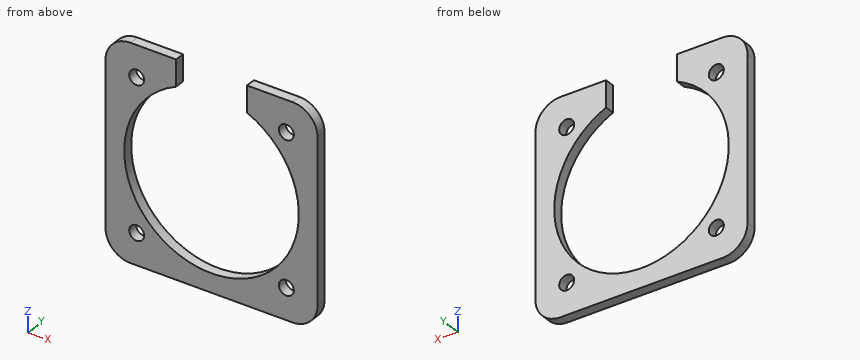
from build123d import *

# Parameters (mm, degrees)
SKETCH1_W           = 40.5
SKETCH1_H           = 40.5
SKETCH1_R           = 17.5
BOSS_EXTRUDE1_DEPTH = 2
SKETCH2_R           = 1.25
CUT_EXTRUDE1_DEPTH  = 2
CUT_EXTRUDE2_DEPTH  = 2
SKETCH4_W           = 42.5
SKETCH4_H           = 42.5
SKETCH4_W_2         = 40.5
SKETCH4_H_2         = 40.5
BOSS_EXTRUDE2_DEPTH = 2
SKETCH5_W           = 14.2
SKETCH5_H           = 2
CUT_EXTRUDE3_DEPTH  = 2
SKETCH6_R           = 1.5
CUT_EXTRUDE4_DEPTH  = 3.5
SKETCH7_R           = 1.5
BOSS_EXTRUDE3_DEPTH = 2
SKETCH8_R           = 1.5
CUT_EXTRUDE5_DEPTH  = 2
FILLET2_R           = 5


with BuildPart() as part:
    # Sketch1 → Boss-Extrude1 (new body)
    with BuildSketch(Plane(origin=(0, 0, 0), x_dir=(1, 0, 0), z_dir=(0, 1, 0))):
        Rectangle(SKETCH1_W, SKETCH1_H)
        with Locations(Location((0, 0, 0), (0, 0, 270))):
            Circle(SKETCH1_R, mode=Mode.SUBTRACT)
    extrude(amount=BOSS_EXTRUDE1_DEPTH)

    # Sketch2 → Cut-Extrude1 (cut)
    with BuildSketch(Plane(origin=(0, 2, 0), x_dir=(1, 0, 0), z_dir=(0, 1, 0))):
        with Locations(Location((-15, 15, 0), (0, 0, 270))):
            Circle(SKETCH2_R)
        with Locations(Location((15, 15, 0), (0, 0, 270))):
            Circle(SKETCH2_R)
        with Locations(Location((-15, -15, 0), (0, 0, 270))):
            Circle(SKETCH2_R)
        with Locations(Location((15, -16.25, 0), (0, 0, 270))):
            Circle(SKETCH2_R)
    extrude(amount=-CUT_EXTRUDE1_DEPTH, mode=Mode.SUBTRACT)

    # Sketch3 → Cut-Extrude2 (cut)
    with BuildSketch(Plane(origin=(0, 2, 0), x_dir=(1, 0, 0), z_dir=(0, 1, 0))):
        Polygon((0, -20.25), (7.1, -20.25), (7.1, -15.994999219), (-7.1, -15.994999219), (-7.1, -20.25), align=None)
    extrude(amount=-CUT_EXTRUDE2_DEPTH, mode=Mode.SUBTRACT)

    # Sketch4 → Boss-Extrude2 (add)
    with BuildSketch(Plane(origin=(0, 2, 0), x_dir=(1, 0, 0), z_dir=(0, 1, 0))):
        Rectangle(SKETCH4_W, SKETCH4_H)
        Rectangle(SKETCH4_W_2, SKETCH4_H_2, mode=Mode.SUBTRACT)
    extrude(amount=-BOSS_EXTRUDE2_DEPTH)

    # Sketch5 → Cut-Extrude3 (cut)
    with BuildSketch(Plane(origin=(0, 2, 0), x_dir=(1, 0, 0), z_dir=(0, 1, 0))):
        with Locations((0, -21.25)):
            Rectangle(SKETCH5_W, SKETCH5_H)
    extrude(amount=-CUT_EXTRUDE3_DEPTH, mode=Mode.SUBTRACT)

    # Sketch6 → Cut-Extrude4 (cut)
    with BuildSketch(Plane(origin=(0, 2, 0), x_dir=(1, 0, 0), z_dir=(0, 1, 0))):
        with Locations(Location((-15, 15, 0), (0, 0, 270))):
            Circle(SKETCH6_R)
        with Locations(Location((15, 15, 0), (0, 0, 270))):
            Circle(SKETCH6_R)
        with Locations(Location((15, -16.25, 0), (0, 0, 270))):
            Circle(SKETCH6_R)
        with Locations(Location((-15, -15, 0), (0, 0, 270))):
            Circle(SKETCH6_R)
    extrude(amount=-CUT_EXTRUDE4_DEPTH, mode=Mode.SUBTRACT)

    # Sketch7 → Boss-Extrude3 (add)
    with BuildSketch(Plane(origin=(0, 2, 0), x_dir=(1, 0, 0), z_dir=(0, 1, 0))):
        with Locations((15, -16.25)):
            Circle(SKETCH7_R)
    extrude(amount=-BOSS_EXTRUDE3_DEPTH)

    # Sketch8 → Cut-Extrude5 (cut)
    with BuildSketch(Plane(origin=(0, 2, 0), x_dir=(1, 0, 0), z_dir=(0, 1, 0))):
        with Locations(Location((15, -15, 0), (0, 0, 270))):
            Circle(SKETCH8_R)
    extrude(amount=-CUT_EXTRUDE5_DEPTH, mode=Mode.SUBTRACT)

    # Fillet2
    fillet2_edges = [part.edges().sort_by_distance(p)[0] for p in [
        (-21.25, 1, 21.25),
        (-21.25, 1, -21.25),
        (21.25, 1, -21.25),
        (21.25, 1, 21.25),
    ]]
    fillet(fillet2_edges, radius=FILLET2_R)


solid = part.part
Source: CAD feature listing. Evaluate the final solid. Frame: model axes, mm. Round coordinates to 2 decimals unless told otherwise and drop trailing zeros. Loops run counter-clockwise (first coordinate to the right, second up) from the corner with the lowest first, then second, coordinate; pieces in that order, holes last. Notation, with made-up numbers: (-20, -28) - (-8, -28) arc R10 ccw to (-8, -16) - close; hole circle Ø3 at (67, 66.25). An arc over 180 degrees is marked (long way). Write item = value, one per line. Start each with the question number.
Item 1: Section query C-C on x = 12. Output: boundary loops of the cut face in (y, z).
Item 2: First-contact query: pin 1 Ø0.6 at (y, z) = (1, 19.5) entering from -X; pin 2 Ø1.8 at (x, z) = (-15, 15) entering from +Y; pin 3 Ø4 at (x, z) = (15, 15) entering from -Y. Flat tips, straight axial feed; report the tip coordinate or a pass-through.
Item 3: Section query D-D on z = -15. Output: boundary loops of the cut face in (x, y).
Item 4: Section query A-A on z = 0. Output: boundary loops of the cut face in (x, y).
Item 5: Section query B-B on y = 0.35. Output: boundary loops of the cut face in (x, z) (3 decimals), plus the area to 3 significant figures.
Item 6: Material intervals for line 1 (X direction, y = 0.55, z = 15); line 2 (Z direction, x = 16, y = 1.45); line 3 (X direction, y = 1.35, z = 6.5), sorted ascending.
Results list:
q1.outline = (0, -21.25) - (2, -21.25) - (2, -12.74) - (0, -12.74) - close; (0, 12.74) - (2, 12.74) - (2, 21.25) - (0, 21.25) - close
q2.pin_1 = -20.29
q2.pin_2 = through
q2.pin_3 = 0
q3.outline = (-21.25, 0) - (-16.5, 0) - (-16.5, 2) - (-21.25, 2) - close; (-13.5, 0) - (-9.01, 0) - (-9.01, 2) - (-13.5, 2) - close; (9.01, 0) - (13.5, 0) - (13.5, 2) - (9.01, 2) - close; (16.5, 0) - (21.25, 0) - (21.25, 2) - (16.5, 2) - close
q4.outline = (-21.25, 0) - (-17.5, 0) - (-17.5, 2) - (-21.25, 2) - close; (17.5, 0) - (21.25, 0) - (21.25, 2) - (17.5, 2) - close
q5.outline = (-21.25, -16.25) arc R5 ccw to (-16.25, -21.25) - (16.25, -21.25) arc R5 ccw to (21.25, -16.25) - (21.25, 16.25) arc R5 ccw to (16.25, 21.25) - (7.1, 21.25) - (7.1, 15.995) arc R17.5 cw (long way) to (-7.1, 15.995) - (-7.1, 21.25) - (-16.25, 21.25) arc R5 ccw to (-21.25, 16.25) - close; hole circle Ø3 at (-15, -15); hole circle Ø3 at (-15, 15); hole circle Ø3 at (15, -15); hole circle Ø3 at (15, 15)
q5.area = 734 mm²
q6.line_1 = -21.25 to -16.5, -13.5 to -9.01, 9.01 to 13.5, 16.5 to 21.25
q6.line_2 = -21.25 to -16.12, -13.88 to -7.09, 7.09 to 13.88, 16.12 to 21.25
q6.line_3 = -21.25 to -16.25, 16.25 to 21.25
